Verification items for the finished model (mm, model axes). Face numbers are marked on the shaded views. A direction names the side the tool comes from. Coordinates: 2 decimals unless noted, no trailing zeros. Order: outer loops, then holes, each group sorted by start corner. A loop starts at its lowest first (then second) coordinate and runs counter-clockwise, first axis right, second up. Notation, with made-up numbers: M 76.25,51.25 L 135.25,51.25 A24 cw 135.25,68.25 Z; hole C -4.5,61 d4. An arc over 180 degrees is marked long. Return JSON: item names as keys, results as strings.
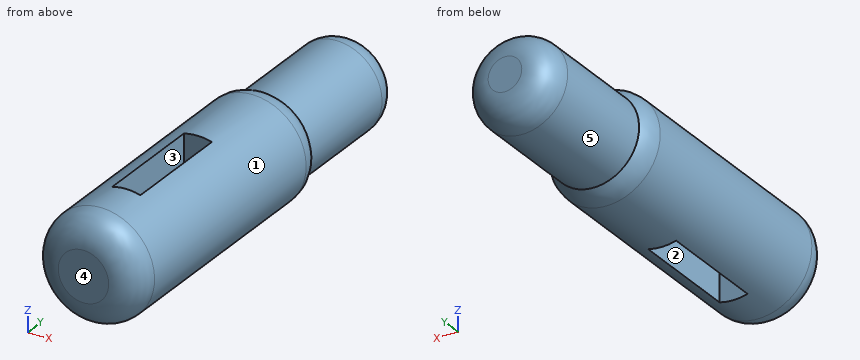
```python
from build123d import *

# Parameters (mm, degrees)
SKETCH1_R               = 19
BOSS_EXTRUDE3_DEPTH     = 102
SKETCH2_R               = 16
BOSS_EXTRUDE4_DEPTH     = 50
FILLET1_R               = 10
FILLET2_R               = 10
FILLET3_R               = 10
CUT_EXTRUDE1_DEPTH      = 155.356729713
CUT_EXTRUDE1_DEPTH_BACK = 155.356729713
SKETCH3_W               = 10
SKETCH3_H               = 40


with BuildPart() as part:
    # Sketch1 → Boss-Extrude3 (new body)
    with BuildSketch(Plane(origin=(0, 0, 0), x_dir=(1, 0, 0), z_dir=(0, 1, 0))):
        with Locations(Location((0, 0, 0), (0, 0, 270))):
            Circle(SKETCH1_R)
    extrude(amount=BOSS_EXTRUDE3_DEPTH)

    # Sketch2 → Boss-Extrude4 (add)
    with BuildSketch(Plane(origin=(0, 102, 0), x_dir=(1, 0, 0), z_dir=(0, 1, 0))):
        with Locations(Location((0, 0, 0), (0, 0, 270))):
            Circle(SKETCH2_R)
    extrude(amount=BOSS_EXTRUDE4_DEPTH)

    # Fillet1
    # the kernel refuses this fillet: 10 mm, written as the material it takes off along each edge
    with BuildSketch(Plane(origin=(0, 102, 0), x_dir=(0, 0, 1), z_dir=(-1, 0, 0))) as fillet1_piece_1:
        with BuildLine():
            CenterArc((9, -7.141428429), FILLET1_R, 0, 45.572995999)
            Line((16, 0), (16.14, 0.142828569))
            ThreePointArc((16.14, 0.142828569), (17.5, 0.2), (19, 0.2))
            Line((19, 0.2), (19.2, 0))
            Line((19.2, 0), (19.2, -7.141428429))
            Line((19.2, -7.141428429), (19, -7.141428429))
        make_face()
    revolve(axis=Axis((0, 102, 0), (0, 1, 0)), mode=Mode.SUBTRACT)

    # Fillet2
    fillet2_edges = [part.edges().sort_by_distance(p)[0] for p in [
        (0, 152, -16),
    ]]
    fillet(fillet2_edges, radius=FILLET2_R)

    # Fillet3
    fillet3_edges = [part.edges().sort_by_distance(p)[0] for p in [
        (0, 0, -19),
    ]]
    fillet(fillet3_edges, radius=FILLET3_R)

    # Sketch3 → Cut-Extrude1 (cut, two sides: drawn at the far end of the back side and taken through both)
    with BuildSketch(Plane.XY.offset(-CUT_EXTRUDE1_DEPTH_BACK)):
        with Locations((0, 44)):
            Rectangle(SKETCH3_W, SKETCH3_H)
    extrude(amount=CUT_EXTRUDE1_DEPTH + CUT_EXTRUDE1_DEPTH_BACK, mode=Mode.SUBTRACT)


solid = part.part
```
Q1. Draft check along X on the marked faces 3, 4 and 5. Enter one of: pulls with the +X half, pulls with the -X half, needs draft (parallel to the pull), parting line crosses it, or undercut.
Values:
{"face 3": "undercut", "face 4": "needs draft", "face 5": "parting line crosses it"}
Q2. Tool access check on the marked faces 1 and 2. Record the directions out of +Z, -Z, +X, -X, +Y, -Y that give a thin tool (end or side, any length) a straight path to the whole face; none if there is none.
Values:
{"face 1": "+Y, -Y", "face 2": "+Z, -Z"}
Q3. Cross-section at A-A, the plane y = 41. Record the boundary of the cut face in (x, z).
Values:
{"outline": "M -5,-18.33 L -5,18.33 A19 ccw Z; M 5,-18.33 A19 ccw 5,18.33 Z"}
Q4. Cross-section at B-B, the plane y = 139. Record the boundary of the cut face in (x, z), and give its area (3 significant figures).
Values:
{"outline": "C 0,0 d32", "area": "804 mm^2"}
Q5. Go/stop test with flat-tipped pins: pin 1 (8 mm diameter, centred on y = 111.5, z = 7, fed in from -X); pin 2 (1 mm diameter, centred on y = 130, z = 11.5, fed in from +X); pin 3 (10 mm diameter, centred on x = -13.5, z = -11, fed in from +Y). Record where each tip stops, or that it passes through.
Values:
{"pin 1": "x = -15.72", "pin 2": "x = 11.62", "pin 3": "y = 149.67"}
Q6. Material ranges on line 1 along X through (y, z) = (42, -5); line 2 along X through (y, z) = (61, 7); line 3 along Y through (x, z) = (-16, -4), recorded low to high.
Values:
{"line 1": "-18.33 to -5, 5 to 18.33", "line 2": "-17.66 to -5, 5 to 17.66", "line 3": "3.38 to 101.48"}
